```python
from build123d import *

# Parameters (mm, degrees)
SKETCH1_W           = 34.417
SKETCH1_H           = 177.8
BOSS_EXTRUDE1_DEPTH = 60.071
FILLET1_R           = 1.27
FILLET2_R           = 1.27
BOSS_EXTRUDE2_DEPTH = 2.54


with BuildPart() as part:
    # Sketch1 → Boss-Extrude1 (new body)
    with BuildSketch(Plane(origin=(0, 0, 0), x_dir=(1, 0, 0), z_dir=(0, 1, 0))):
        Rectangle(SKETCH1_W, SKETCH1_H)
    extrude(amount=BOSS_EXTRUDE1_DEPTH)

    # Fillet1
    fillet1_edges = [part.edges().sort_by_distance(p)[0] for p in [
        (17.2085, 60.071, 0),
        (0, 60.071, -88.9),
        (-17.2085, 60.071, 0),
        (0, 0, -88.9),
        (17.2085, 0, 0),
        (0, 0, 88.9),
        (-17.2085, 0, 0),
        (0, 60.071, 88.9),
    ]]
    fillet(fillet1_edges, radius=FILLET1_R)

    # Fillet2
    # the kernel refuses this fillet: 1.27 mm, written as the material it takes off along each edge
    with BuildSketch(Plane(origin=(-15.9385, 1.27, -87.63), x_dir=(0, 0, -1), z_dir=(-1, 0, 0))) as fillet2_piece_1_section:
        Polygon((0, 0), (FILLET2_R * 1.02, 0), (FILLET2_R * 1.02, FILLET2_R * 1.02), (0, FILLET2_R * 1.02), align=None)
    fillet2_piece_1 = extrude(amount=FILLET2_R * 1.02, mode=Mode.PRIVATE)
    fillet2_piece_1 = fillet2_piece_1 - Plane(origin=(-15.9385, 1.27, -87.63), x_dir=(0, 0.7071067811865475, 0.7071067811865475), z_dir=(-1, 0, 0)) * Sphere(FILLET2_R, mode=Mode.PRIVATE)
    add(fillet2_piece_1, mode=Mode.SUBTRACT)
    with BuildSketch(Plane(origin=(15.9385, 1.27, -87.63), x_dir=(0, 0, -1), z_dir=(1, 0, 0))) as fillet2_piece_2_section:
        Polygon((0, 0), (FILLET2_R * 1.02, 0), (FILLET2_R * 1.02, -FILLET2_R * 1.02), (0, -FILLET2_R * 1.02), align=None)
    fillet2_piece_2 = extrude(amount=FILLET2_R * 1.02, mode=Mode.PRIVATE)
    fillet2_piece_2 = fillet2_piece_2 - Plane(origin=(15.9385, 1.27, -87.63), x_dir=(0, 0.7071067811865475, 0.7071067811865475), z_dir=(1, 0, 0)) * Sphere(FILLET2_R, mode=Mode.PRIVATE)
    add(fillet2_piece_2, mode=Mode.SUBTRACT)
    with BuildSketch(Plane(origin=(-15.9385, 1.27, 87.63), x_dir=(-1, 0, 0), z_dir=(0, 0, 1))) as fillet2_piece_3_section:
        Polygon((0, 0), (FILLET2_R * 1.02, 0), (FILLET2_R * 1.02, FILLET2_R * 1.02), (0, FILLET2_R * 1.02), align=None)
    fillet2_piece_3 = extrude(amount=FILLET2_R * 1.02, mode=Mode.PRIVATE)
    fillet2_piece_3 = fillet2_piece_3 - Plane(origin=(-15.9385, 1.27, 87.63), x_dir=(0.7071067811865475, 0.7071067811865475, 0), z_dir=(0, 0, 1)) * Sphere(FILLET2_R, mode=Mode.PRIVATE)
    add(fillet2_piece_3, mode=Mode.SUBTRACT)
    with BuildSketch(Plane(origin=(15.9385, 1.27, 87.63), x_dir=(1, 0, 0), z_dir=(0, 0, 1))) as fillet2_piece_4_section:
        Polygon((0, 0), (FILLET2_R * 1.02, 0), (FILLET2_R * 1.02, -FILLET2_R * 1.02), (0, -FILLET2_R * 1.02), align=None)
    fillet2_piece_4 = extrude(amount=FILLET2_R * 1.02, mode=Mode.PRIVATE)
    fillet2_piece_4 = fillet2_piece_4 - Plane(origin=(15.9385, 1.27, 87.63), x_dir=(-0.7071067811865475, 0.7071067811865475, 0), z_dir=(0, 0, 1)) * Sphere(FILLET2_R, mode=Mode.PRIVATE)
    add(fillet2_piece_4, mode=Mode.SUBTRACT)
    with BuildSketch(Plane(origin=(15.9385, 58.801, 87.63), x_dir=(1, 0, 0), z_dir=(0, 0, 1))) as fillet2_piece_5_section:
        Polygon((0, 0), (FILLET2_R * 1.02, 0), (FILLET2_R * 1.02, FILLET2_R * 1.02), (0, FILLET2_R * 1.02), align=None)
    fillet2_piece_5 = extrude(amount=FILLET2_R * 1.02, mode=Mode.PRIVATE)
    fillet2_piece_5 = fillet2_piece_5 - Plane(origin=(15.9385, 58.801, 87.63), x_dir=(-0.7071067811865475, -0.7071067811865475, 0), z_dir=(0, 0, 1)) * Sphere(FILLET2_R, mode=Mode.PRIVATE)
    add(fillet2_piece_5, mode=Mode.SUBTRACT)
    with BuildSketch(Plane(origin=(-15.9385, 58.801, 87.63), x_dir=(-1, 0, 0), z_dir=(0, 0, 1))) as fillet2_piece_6_section:
        Polygon((0, 0), (FILLET2_R * 1.02, 0), (FILLET2_R * 1.02, -FILLET2_R * 1.02), (0, -FILLET2_R * 1.02), align=None)
    fillet2_piece_6 = extrude(amount=FILLET2_R * 1.02, mode=Mode.PRIVATE)
    fillet2_piece_6 = fillet2_piece_6 - Plane(origin=(-15.9385, 58.801, 87.63), x_dir=(0.7071067811865475, -0.7071067811865475, 0), z_dir=(0, 0, 1)) * Sphere(FILLET2_R, mode=Mode.PRIVATE)
    add(fillet2_piece_6, mode=Mode.SUBTRACT)
    with BuildSketch(Plane(origin=(15.9385, 58.801, -87.63), x_dir=(0, 0, -1), z_dir=(1, 0, 0))) as fillet2_piece_7_section:
        Polygon((0, 0), (FILLET2_R * 1.02, 0), (FILLET2_R * 1.02, FILLET2_R * 1.02), (0, FILLET2_R * 1.02), align=None)
    fillet2_piece_7 = extrude(amount=FILLET2_R * 1.02, mode=Mode.PRIVATE)
    fillet2_piece_7 = fillet2_piece_7 - Plane(origin=(15.9385, 58.801, -87.63), x_dir=(0, -0.7071067811865475, 0.7071067811865475), z_dir=(1, 0, 0)) * Sphere(FILLET2_R, mode=Mode.PRIVATE)
    add(fillet2_piece_7, mode=Mode.SUBTRACT)
    with BuildSketch(Plane(origin=(-15.9385, 58.801, -87.63), x_dir=(0, 0, -1), z_dir=(-1, 0, 0))) as fillet2_piece_8_section:
        Polygon((0, 0), (FILLET2_R * 1.02, 0), (FILLET2_R * 1.02, -FILLET2_R * 1.02), (0, -FILLET2_R * 1.02), align=None)
    fillet2_piece_8 = extrude(amount=FILLET2_R * 1.02, mode=Mode.PRIVATE)
    fillet2_piece_8 = fillet2_piece_8 - Plane(origin=(-15.9385, 58.801, -87.63), x_dir=(0, -0.7071067811865475, 0.7071067811865475), z_dir=(-1, 0, 0)) * Sphere(FILLET2_R, mode=Mode.PRIVATE)
    add(fillet2_piece_8, mode=Mode.SUBTRACT)
    with BuildSketch(Plane(origin=(17.2085, 1.27, 88.9), x_dir=(-1, 0, 0), z_dir=(0, 1, 0)), Plane(origin=(17.2085, 1.27, -88.9), x_dir=(0, 0, 1), z_dir=(0, 1, 0))) as fillet2_piece_9:
        with BuildLine():
            CenterArc((FILLET2_R, -FILLET2_R), FILLET2_R, 90, 90)
            Line((0, -FILLET2_R), (0, 0))
            Line((0, 0), (FILLET2_R, 0))
        make_face()
    extrude(amount=57.531, mode=Mode.SUBTRACT)
    with BuildSketch(Plane(origin=(-17.2085, 1.27, 88.9), x_dir=(1, 0, 0), z_dir=(0, 1, 0)), Plane(origin=(-17.2085, 1.27, -88.9), x_dir=(0, 0, 1), z_dir=(0, 1, 0))) as fillet2_piece_10:
        with BuildLine():
            CenterArc((FILLET2_R, FILLET2_R), FILLET2_R, 180, 90)
            Line((0, FILLET2_R), (0, 0))
            Line((0, 0), (FILLET2_R, 0))
        make_face()
    extrude(amount=57.531, mode=Mode.SUBTRACT)

    # Sketch2 → Boss-Extrude2 (add, symmetric)
    with BuildSketch(Plane(origin=(0, 0, 0), x_dir=(0, 0, -1), z_dir=(1, 0, 0))):
        with BuildLine():
            Line((-82.55, 60.071), (-82.55, 62.103))
            ThreePointArc((-82.55, 62.103), (-82.401210245, 62.462210245), (-82.042, 62.611))
            Line((-82.042, 62.611), (-77.978, 62.611))
            ThreePointArc((-77.978, 62.611), (-77.618789755, 62.462210245), (-77.47, 62.103))
            Line((-77.47, 62.103), (-77.47, 61.849))
            ThreePointArc((-77.47, 61.849), (-77.618789755, 61.489789755), (-77.978, 61.341))
            Line((-77.978, 61.341), (-80.772, 61.341))
            ThreePointArc((-80.772, 61.341), (-81.131210245, 61.192210245), (-81.28, 60.833))
            Line((-81.28, 60.833), (-81.28, 60.071))
            Line((-81.28, 60.071), (-82.55, 60.071))
        make_face()
    boss_extrude2 = extrude(amount=BOSS_EXTRUDE2_DEPTH, both=True)

    # Mirror1: Boss-Extrude2 across plane
    add(boss_extrude2.mirror(Plane.XY))


solid = part.part
```
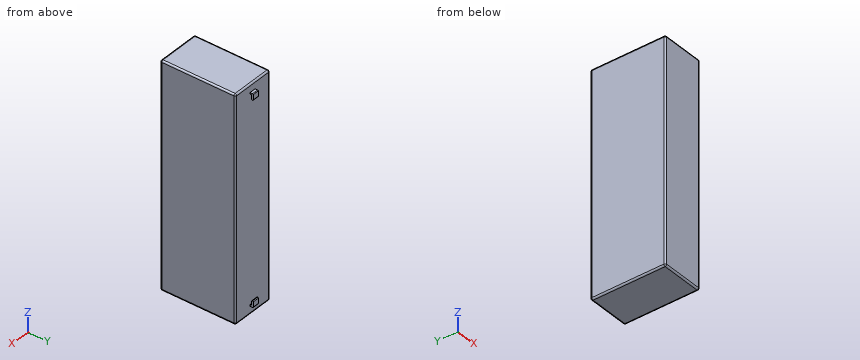
Geometry check sheet. Reference: the model listing, model coordinates, mm. Give positions to 0.01 mm unless a question says otherwise; leave off trailing zeros. Write each loop counter-clockwise with the first axis right and the second up, starting at its lowest first coordinate (ties: lowest second). Pieces come first, ordered by that corner, then holes.
1) Section check B-B, the plane z = -26.5. Record the boundary of the cut face in (x, y).
2) Section check C-C, the plane x = -12. Record the boundary of the cut face in (y, z).
3) Gauge pin test, flat ends, axial feed: pin 1 (9.5 mm diameter, centred on x = 4, z = 33.5, fed in from +Y); pin 2 (0.8 mm diameter, centred on y = 61, z = -79, fed in from +X); pin 3 (1.6 mm diameter, centred on x = 1, y = 61.5, fed in from +Z). Record the tip position at first contact, or that the pin passes through.
4) Section check A-A, the plane x = -0.5. Record the boundary of the cut face in (y, z).
5) Material ranges on L1, parallel to X at y = 59, z = -3; L2, parallel to Y at x = 1.5, z = 7.5, recorded low to high.
Computed:
1. outline: (-17.21, 1.27) arc R1.27 ccw to (-15.94, 0) - (15.94, 0) arc R1.27 ccw to (17.21, 1.27) - (17.21, 58.8) arc R1.27 ccw to (15.94, 60.07) - (-15.94, 60.07) arc R1.27 ccw to (-17.21, 58.8) - close
2. outline: (0, -87.63) arc R1.27 ccw to (1.27, -88.9) - (58.8, -88.9) arc R1.27 ccw to (60.07, -87.63) - (60.07, 87.63) arc R1.27 ccw to (58.8, 88.9) - (1.27, 88.9) arc R1.27 ccw to (0, 87.63) - close
3. pin 1: stops at y = 60.07
3. pin 2: stops at x = 2.54
3. pin 3: stops at z = 82.55
4. outline: (0, -87.63) arc R1.27 ccw to (1.27, -88.9) - (58.8, -88.9) arc R1.27 ccw to (60.07, -87.63) - (60.07, -82.55) - (62.1, -82.55) arc R0.51 ccw to (62.61, -82.04) - (62.61, -77.98) arc R0.51 ccw to (62.1, -77.47) - (61.85, -77.47) arc R0.51 ccw to (61.34, -77.98) - (61.34, -80.77) arc R0.51 cw to (60.83, -81.28) - (60.07, -81.28) - (60.07, 81.28) - (60.83, 81.28) arc R0.51 cw to (61.34, 80.77) - (61.34, 77.98) arc R0.51 ccw to (61.85, 77.47) - (62.1, 77.47) arc R0.51 ccw to (62.61, 77.98) - (62.61, 82.04) arc R0.51 ccw to (62.1, 82.55) - (60.07, 82.55) - (60.07, 87.63) arc R1.27 ccw to (58.8, 88.9) - (1.27, 88.9) arc R1.27 ccw to (0, 87.63) - close
5. L1: x = -17.19 to 17.19
5. L2: y = 0 to 60.07
